from build123d import *

# Parameters (mm, degrees)
F0_R     = 2.5908
F3_DEPTH = 31.75
F1_R     = 2.8448
F4_DEPTH = 27.94
F2_R     = 3.0353
F5_DEPTH = 20.32


with BuildPart() as f3:
    # F0 (on Front) → F3 (new body)
    with BuildSketch(Plane.XZ):
        Circle(F0_R)
    extrude(amount=F3_DEPTH)

    # F1 (on Front) → F4 (join)
    with BuildSketch(Plane.XZ):
        Circle(F1_R)
    extrude(amount=F4_DEPTH)

    # F2 (on Front) → F5 (join)
    with BuildSketch(Plane.XZ):
        Circle(F2_R)
    extrude(amount=F5_DEPTH)


solid = f3.part
Could you check a few things on this model? Use its own coordinates, in mm. A direction names the side the tool comes from. Give positions to 0.01 mm unless a question says otherwise; leave off trailing zeros. Order: outer loops, then holes, each group sorted by start corner. A loop starts at its lowest first (then second) coordinate and runs counter-clockwise, first axis right, second up.
1. Suppose I cut it at C-C (y = -12). List the corners of the cut face in (x, z) for me.
2. For faces 1 (the flat face through (0, 0, 0)), 2 (the cylindrical face through (-0.617, -24.077, -2.777)), which set-ups out of +Z, -Z, +X, -X, +Y, -Y let a thin tool reach every point of the face, with its end or its side?
3. Suppose I cut it at A-A (x = 0). List the corners of the cut face in (y, z) for me, plus the area to 3 significant figures.
4. Suppose I cut it at B-B (z = 0). List the corners of the cut face in (x, y) for me, plus the area to 3 significant figures.
5. Will these pins go through, and if not, where does the flat tip stop? P1, Ø3, axis at x = 0.5, y = -16.5, coming from the +Z side; P2, Ø1.5, axis at y = -15.5, z = 1.5, coming from the +X side.
6. Suppose I cut it at D-D (y = -21). List the corners of the cut face in (x, z) for me.
7. I need wall thicknesses on L1, parallel to Y at x = -2.5, z = 1.25; L2, parallel to Y at x = -2.25, z = -2; L3, parallel to X at y = -29, z = 0. Which ranges of each line are inside material? Lowest first, please.
Solved:
1. outline: circle Ø6.07 at (0, 0)
2. face 1: +Z, -Z, +X, -X, +Y
2. face 2: -Y
3. outline: (-31.75, -2.59) - (-27.94, -2.59) - (-27.94, -2.84) - (-20.32, -2.84) - (-20.32, -3.04) - (0, -3.04) - (0, 3.04) - (-20.32, 3.04) - (-20.32, 2.84) - (-27.94, 2.84) - (-27.94, 2.59) - (-31.75, 2.59) - close
3. area: 186 mm2
4. outline: (-3.04, -20.32) - (-2.84, -20.32) - (-2.84, -27.94) - (-2.59, -27.94) - (-2.59, -31.75) - (2.59, -31.75) - (2.59, -27.94) - (2.84, -27.94) - (2.84, -20.32) - (3.04, -20.32) - (3.04, 0) - (-3.04, 0) - close
4. area: 186 mm2
5. P1: stops at z = 3.04
5. P2: stops at x = 2.94
6. outline: circle Ø5.69 at (0, 0)
7. L1: y = -27.94 to 0
7. L2: y = -20.32 to 0
7. L3: x = -2.59 to 2.59
